from build123d import *

# Parameters (mm, degrees)
SKETCH1_W               = 100
SKETCH1_H               = 60
BOSS_EXTRUDE1_DEPTH     = 10
BOSS_EXTRUDE2_START     = 10
SKETCH3_R               = 22.5
BOSS_EXTRUDE2_DEPTH     = 12
CUT_EXTRUDE2_START      = 22
SKETCH4_R               = 15
CUT_EXTRUDE2_DEPTH      = 14
SKETCH6_W               = 100
SKETCH6_H               = 11.9
BOSS_EXTRUDE3_DEPTH     = 2
CUT_EXTRUDE1_DEPTH      = 63.321745804
CUT_EXTRUDE1_DEPTH_BACK = 63.321745804
SKETCH2_R               = 3.2
CUT_EXTRUDE3_DEPTH      = 63.321745804
CUT_EXTRUDE3_DEPTH_BACK = 63.321745804
SKETCH5_R               = 7.5
CUT_EXTRUDE4_START      = 10
SKETCH8_R               = 5.5
CUT_EXTRUDE4_DEPTH      = 5
CHAMFER1_SIZE           = 5
CHAMFER2_SIZE           = 3
CHAMFER3_SIZE           = 0.8


with BuildPart() as part:
    # Sketch1 → Boss-Extrude1 (new body)
    with BuildSketch(Plane(origin=(0, 0, 0), x_dir=(1, 0, 0), z_dir=(0, 1, 0))):
        Rectangle(SKETCH1_W, SKETCH1_H)
    extrude(amount=BOSS_EXTRUDE1_DEPTH)

    # Sketch3 → Boss-Extrude2 (add)
    with BuildSketch(Plane(origin=(0, 0, 0), x_dir=(1, 0, 0), z_dir=(0, 1, 0)).offset(BOSS_EXTRUDE2_START)):
        with Locations(Location((0, 0, 0), (0, 0, 90))):
            Circle(SKETCH3_R)
    extrude(amount=BOSS_EXTRUDE2_DEPTH)

    # Sketch4 → Cut-Extrude2 (cut)
    with BuildSketch(Plane(origin=(0, 0, 0), x_dir=(1, 0, 0), z_dir=(0, 1, 0)).offset(CUT_EXTRUDE2_START)):
        with Locations(Location((0, 0, 0), (0, 0, 90))):
            Circle(SKETCH4_R)
    extrude(amount=-CUT_EXTRUDE2_DEPTH, mode=Mode.SUBTRACT)

    # Sketch6 → Boss-Extrude3 (add)
    with BuildSketch(Plane(origin=(0, 0, 0), x_dir=(1, 0, 0), z_dir=(0, 1, 0))):
        Rectangle(SKETCH6_W, SKETCH6_H)
    extrude(amount=-BOSS_EXTRUDE3_DEPTH)

    # Sketch2 → Cut-Extrude1 (cut, two sides: drawn at the far end of the back side and taken through both)
    with BuildSketch(Plane(origin=(0, 0, 0), x_dir=(1, 0, 0), z_dir=(0, 1, 0)).offset(-CUT_EXTRUDE1_DEPTH_BACK)):
        with Locations(Location((-40, 0, 0), (0, 0, 90))):
            Circle(SKETCH2_R)
        with Locations(Location((40, 0, 0), (0, 0, 90))):
            Circle(SKETCH2_R)
    extrude(amount=CUT_EXTRUDE1_DEPTH + CUT_EXTRUDE1_DEPTH_BACK, mode=Mode.SUBTRACT)

    # Sketch5 → Cut-Extrude3 (cut, two sides: drawn at the far end of the back side and taken through both)
    with BuildSketch(Plane(origin=(0, 0, 0), x_dir=(1, 0, 0), z_dir=(0, 1, 0)).offset(-CUT_EXTRUDE3_DEPTH_BACK)):
        with Locations(Location((0, 0, 0), (0, 0, 90))):
            Circle(SKETCH5_R)
    extrude(amount=CUT_EXTRUDE3_DEPTH + CUT_EXTRUDE3_DEPTH_BACK, mode=Mode.SUBTRACT)

    # Sketch8 → Cut-Extrude4 (cut)
    with BuildSketch(Plane(origin=(0, 0, 0), x_dir=(1, 0, 0), z_dir=(0, 1, 0)).offset(CUT_EXTRUDE4_START)):
        with Locations(Location((40, 0, 0), (0, 0, 90))):
            Circle(SKETCH8_R)
        with Locations(Location((-40, 0, 0), (0, 0, 90))):
            Circle(SKETCH8_R)
    extrude(amount=-CUT_EXTRUDE4_DEPTH, mode=Mode.SUBTRACT)

    # Chamfer1
    # the kernel refuses this chamfer: 5 mm, written as the material it takes off along each edge
    with BuildSketch(Plane(origin=(-50, 10, -42.85841494), x_dir=(0.9996219169112968, 0.027495876610586317, 0), z_dir=(0, 0, 1)), Plane(origin=(50, 10, 42.85841494), x_dir=(-0.9996219169112968, 0.027495876610586317, 0), z_dir=(0, 0, -1))) as chamfer1_piece_1:
        Polygon((CHAMFER1_SIZE * 0.999621916911, -CHAMFER1_SIZE * 0.0274958766106), (-CHAMFER1_SIZE * 0.0274958766106, -CHAMFER1_SIZE * 0.999621916911), (0, 0), align=None)
    extrude(amount=85.71682988, mode=Mode.SUBTRACT)
    with BuildSketch(Plane(origin=(-62.85841494, 10, 30), x_dir=(0, -0.9996219169112968, 0.027495876610586317), z_dir=(1, 0, 0))) as chamfer1_piece_2:
        Polygon((CHAMFER1_SIZE * 0.999621916911, CHAMFER1_SIZE * 0.0274958766106), (-CHAMFER1_SIZE * 0.0274958766106, CHAMFER1_SIZE * 0.999621916911), (0, 0), align=None)
    extrude(amount=125.71682988, mode=Mode.SUBTRACT)
    with BuildSketch(Plane(origin=(62.85841494, 10, -30), x_dir=(0, 0.027495876610586317, 0.9996219169112968), z_dir=(-1, 0, 0))) as chamfer1_piece_3:
        Polygon((CHAMFER1_SIZE * 0.999621916911, -CHAMFER1_SIZE * 0.0274958766106), (-CHAMFER1_SIZE * 0.0274958766106, -CHAMFER1_SIZE * 0.999621916911), (0, 0), align=None)
    extrude(amount=125.71682988, mode=Mode.SUBTRACT)

    # Chamfer2
    chamfer2_edges = [part.edges().sort_by_distance(p)[0] for p in [
        (0, 22, 22.5),
    ]]
    chamfer(chamfer2_edges, length=CHAMFER2_SIZE)

    # Chamfer3
    chamfer3_edges = [part.edges().sort_by_distance(p)[0] for p in [
        (27.282953131, -2, -5.95),
        (-27.282953131, -2, 5.95),
        (-27.282953131, -2, -5.95),
        (27.282953131, -2, 5.95),
    ]]
    chamfer(chamfer3_edges, length=CHAMFER3_SIZE)


solid = part.part
Work out the finished part from the listing and answer in its coordinate system (mm). A direction names the side the tool comes from. Give positions to 0.01 mm unless a question says otherwise; leave off trailing zeros. Order: outer loops, then holes, each group sorted by start corner. A loop starts at its lowest first (then second) coordinate and runs counter-clockwise, first axis right, second up. Notation, with made-up numbers: (22.25, -27.75) -> (69.25, -27.75) arc R20 cw to (69.25, 5.25) -> close; hole circle Ø9 at (65.5, -31.75). An arc over 180 degrees is marked (long way). One line per item, written item: value.
Item 1: Straight lines are drawn through the part: probe 1 along X at (y, z) = (3, 0); probe 2 along X at (y, z) = (19, 0); probe 3 along X at (y, z) = (-0.5, -1.5). For each, find the intervals that lie inside material, in ascending order.
Answer sheet:
probe 1: -50 to -43.2, -36.8 to -7.5, 7.5 to 36.8, 43.2 to 50
probe 2: -22.5 to -15, 15 to 22.5
probe 3: -50 to -42.83, -37.17 to -7.35, 7.35 to 37.17, 42.83 to 50
Item 2: Find section D-D, the plane x = -29. Give the vertices of the cut face in (y, z), plus the area to 3 significant figures.
Answer sheet:
outline: (-2, -5.15) -> (-1.2, -5.95) -> (0, -5.95) -> (0, -30) -> (5, -30) -> (10, -25) -> (10, 25) -> (5, 30) -> (0, 30) -> (0, 5.95) -> (-1.2, 5.95) -> (-2, 5.15) -> close
area: 598 mm²
Item 3: Find section A-A, the plane x = 0. Give the vertices of the cut face in (y, z), plus the area to 3 significant figures.
Answer sheet:
outline: (0, -30) -> (5, -30) -> (10, -25) -> (10, -22.5) -> (19, -22.5) -> (22, -19.5) -> (22, -15) -> (8, -15) -> (8, -7.5) -> (0, -7.5) -> close; (0, 7.5) -> (8, 7.5) -> (8, 15) -> (22, 15) -> (22, 19.5) -> (19, 22.5) -> (10, 22.5) -> (10, 25) -> (5, 30) -> (0, 30) -> close
area: 566 mm²
Item 4: Flat-ended cylindrical pins translate along their axes: P1, Ø12, axis at x = 28.5, y = 15, coming from the +Z side; P2, Ø1.5, axis at y = 14, z = 20, coming from the -X side; P3, Ø6, axis at x = -3, y = 13.5, coming from the +Z side. Find the tip coordinate at first contact, or state that the pin passes through.
Answer sheet:
P1: z = 26
P2: x = -11.65
P3: z = 22.5
Item 5: Find section C-C, the plane y = 1.5. Give the vertices of the cut face in (x, z).
Answer sheet:
outline: (-50, -30) -> (50, -30) -> (50, 30) -> (-50, 30) -> close; hole circle Ø6.4 at (-40, 0); hole circle Ø15 at (0, 0); hole circle Ø6.4 at (40, 0)
Item 6: A tool of negligible diameter and unlimited length cuts with its end or side. For faces 1 (the cylindrical face through (36.827, 1.451, 0.417)), 2 (the flat face through (42.4, 5, -2.4)), 3 (the flat face through (-1, 2, -30)), 4 (the flat face through (-1, 0, 18)), 5 (the flat face through (-1, 0, -18)), from which of +Z, -Z, +X, -X, +Y, -Y can it reach the whole face along a straight path? Write none if from no direction.
Answer sheet:
face 1: +Y, -Y
face 2: +Y
face 3: -Z, +X, -X, +Y, -Y
face 4: +Z, +X, -X, -Y
face 5: -Z, +X, -X, -Y
Item 7: Determine the mould class of faces 6 (the flat face through (47, 8, 0)), 7 (the flat face through (-1, 7, 28)), 8 (the cylindrical face through (-34.63, 7.54, 1.19)), 9 (the cylindrical face through (8.618, 14.437, -20.784)) for opening direction Z: released by +Z, released by -Z, zero draft, split by the parting line, or undercut.
Answer sheet:
face 6: zero draft
face 7: released by +Z
face 8: undercut
face 9: split by the parting line
Item 8: Find section B-B, the plane z = 0. State how many separate pieces and enclosed holes the cut face has, plus the area to 3 significant figures.
Answer sheet:
separate pieces: 4
enclosed holes: 0
area: 937 mm²
